Geometry: see drawing. Coordinates: mm, zero at the bounding-box minimum. Coordinates: 2 decimals unless noted, no trailing zeros. Order: outer loops, then holes, each group sorted by start corner. A loop starts at its lowest first (then second) coordinate and runs counter-clockwise, first axis right, second up. Notation, with made-up numbers: (87.5, 41) - (132.5, 41) arc R22 ccw to (132.5, 65) - close; hole circle Ø2 at (11, -3). An arc over 180 degrees is marked (long way). Use a Markdown table: item, result. Add a question column.
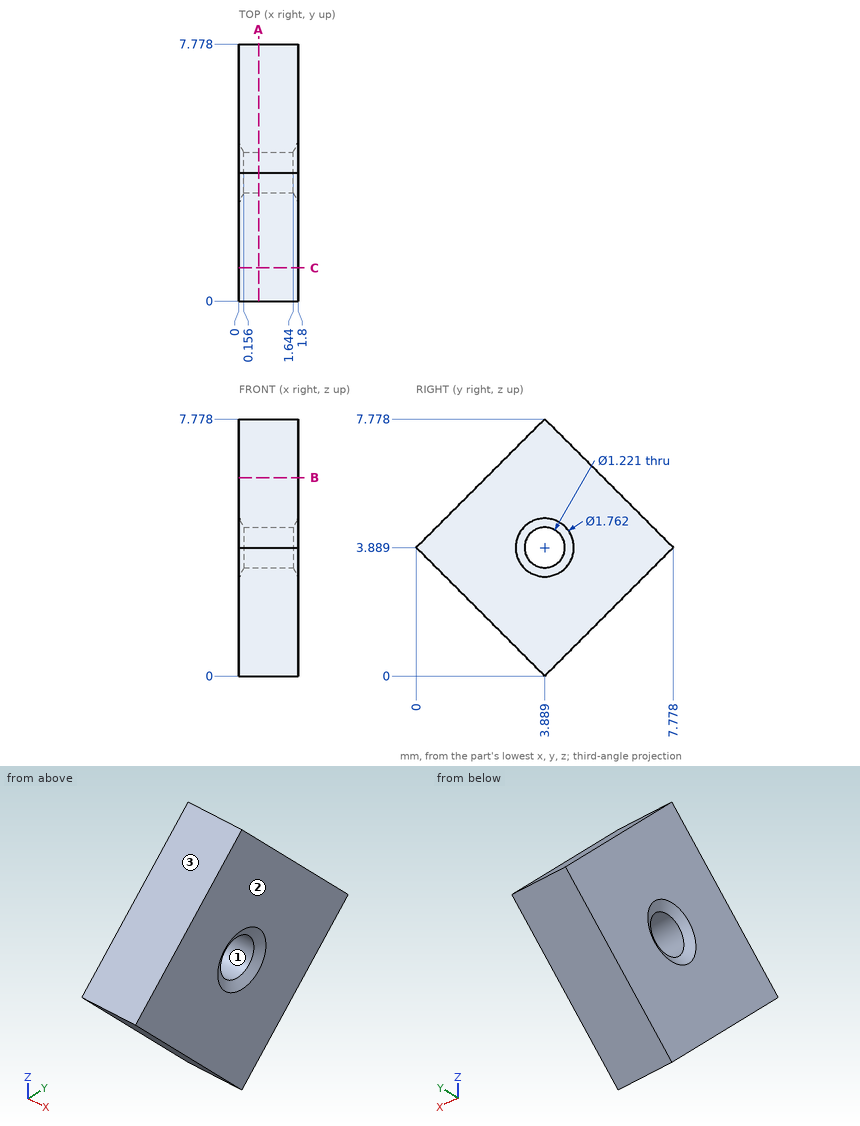
1) Draft query along Z for the marked faces 1, 2 and 3. Return one class per face: released by +Z, released by -Z, zero draft, split by the parting line, or undercut.
2) Section query A-A (x = 0.6). Return the cut outline in (y, z).
3) Line query: line 1 (Z direction, x = 0.95, y = 4.25); line 2 (Y direction, x = 0.85, z = 3.75) (1 decimal); line 3 (Y direction, x = 1.05, z = 2.5). Output: solid intervals per line, ascending. Write a range as from..to.
4) First-contact query: pin 1 (1 mm diameter, centred on x = 1.5, z = 3, fed in from +Y); pin 2 (1.6 mm diameter, centred on y = 3.89, z = 3.89, fed in from -X). Flat tips, straight axial feed; report the tip coordinate or a pass-through.
5) Section query C-C (y = 1). Return the cut outline in (x, z), and give its area (3 significant figures).
6) Section query B-B (z = 6). Return the cut outline in (x, y).
From the geometry:
| question | item | result |
|---|---|---|
| 1 | face 1 | undercut |
| 1 | face 2 | zero draft |
| 1 | face 3 | released by +Z |
| 2 | outline | (0, 3.89) - (3.89, 0) - (7.78, 3.89) - (3.89, 7.78) - close; hole circle Ø1.22 at (3.89, 3.89) |
| 3 | line 1 | z = 0.36..3.4, 4.38..7.42 |
| 3 | line 2 | y = 0.1..3.3, 4.5..7.6 |
| 3 | line 3 | y = 1.39..6.39 |
| 4 | pin 1 | stops at y = 7.39 |
| 4 | pin 2 | stops at x = 0.05 |
| 5 | outline | (0, 2.89) - (1.8, 2.89) - (1.8, 4.89) - (0, 4.89) - close |
| 5 | area | 3.60 mm^2 |
| 6 | outline | (0, 2.11) - (1.8, 2.11) - (1.8, 5.67) - (0, 5.67) - close |
